Drawing for the job (mm, zero at the part's lowest x, y, z). A direction names the side the tool comes from. Give positions to 0.01 mm unless a question says otherwise; leave off trailing zeros. Loops run counter-clockwise (first coordinate to the right, second up) from the corner with the lowest first, then second, coordinate; pieces in that order, holes last. Notation, with made-up numbers: (-32.5, 12) - (2.5, 12) arc R37 cw to (2.5, 51) - close; hole circle Ø3 at (64.25, 51.5). An arc over 180 degrees is marked (long way). Return JSON: item names as keys, results as strings. Group by question number.
1) Slice it at A-A (y = 7.5). List the corners of the cut face in (x, z), and give its area (3 significant figures).
2) Drill centre lines: probe 1 along X at (y, z) = (6, 21); probe 2 along X at (y, z) = (2.2, 12.5); probe 3 along Y at (x, z) = (3, 14.5). Where is each one in solid material? Low to high. Write a range as from..to.
3) Slice it at C-C (x = 4.5). List the corners of the cut face in (y, z), and give its area (3 significant figures).
4) Slice it at D-D (y = 3.25). List the corners of the cut face in (x, z).
5) Drop a flat-ended pin along its axis: pin 1 (2.5 mm diameter, centred on x = 19, z = 12, fed in from +Y). Give the stop position or say it passes through.
6) Slice it at B-B (z = 12.5). List the corners of the cut face in (x, y).
7) 3-axis set-ups, long thin cutter, end or side, ignore diameter. For the marked faces 1 and 2: which of +Z, -Z, +X, -X, +Y, -Y reach the whole face in a straight line?
8) Mould opens along Z. For the marked faces 3, 4, 5 and 6 say: released by +Z, released by -Z, zero draft, split by the parting line, or undercut.
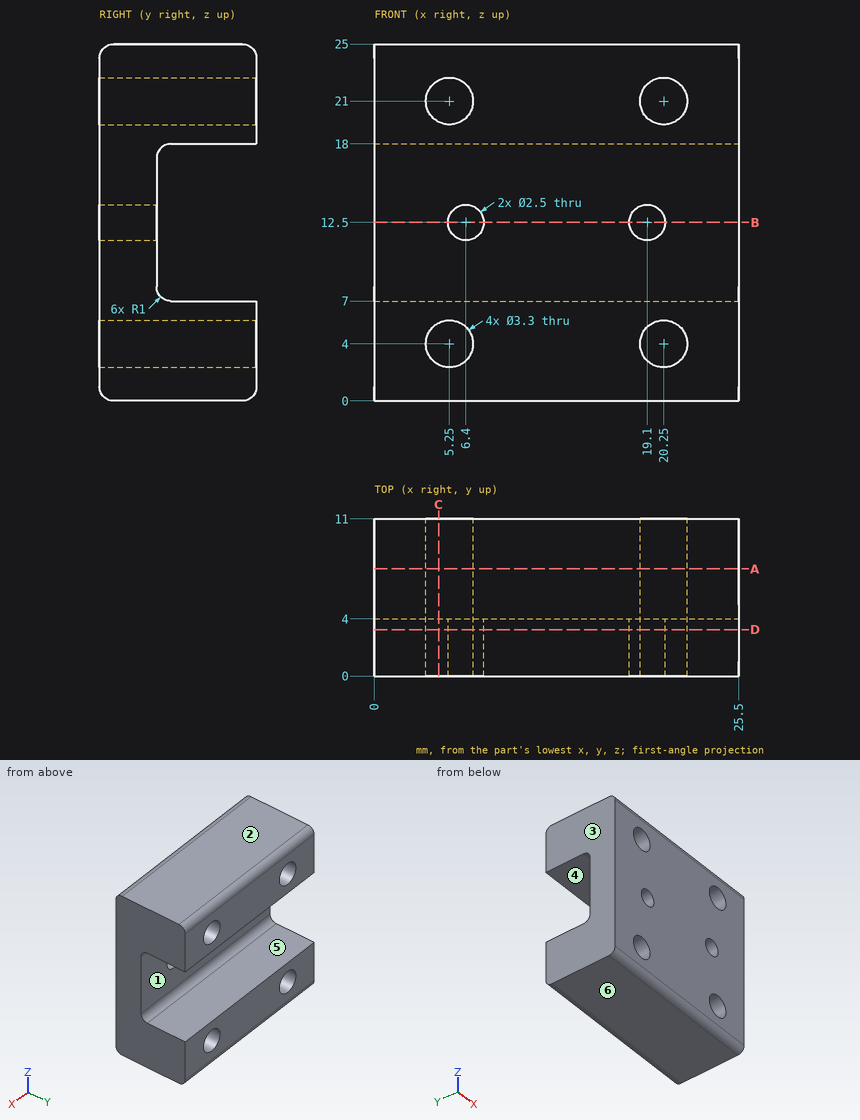
Results:
{
 "1": {"outline": "(0, 0) - (25.5, 0) - (25.5, 7) - (0, 7) - close; (0, 18) - (25.5, 18) - (25.5, 25) - (0, 25) - close; hole circle Ø3.3 at (5.25, 4); hole circle Ø3.3 at (5.25, 21); hole circle Ø3.3 at (20.25, 4); hole circle Ø3.3 at (20.25, 21)", "area": "323 mm2"},
 "2": {"probe 1": "0..3.6, 6.9..18.6, 21.9..25.5", "probe 2": "0..5.15, 7.65..17.85, 20.35..25.5", "probe 3": "0..4"},
 "3": {"outline": "(0, 1) arc R1 ccw to (1, 0) - (10, 0) arc R1 ccw to (11, 1) - (11, 2.53) - (0, 2.53) - close; (0, 5.47) - (11, 5.47) - (11, 7) - (5, 7) arc R1 cw to (4, 8) - (4, 17) arc R1 cw to (5, 18) - (11, 18) - (11, 19.53) - (0, 19.53) - close; (0, 22.47) - (11, 22.47) - (11, 24) arc R1 ccw to (10, 25) - (1, 25) arc R1 ccw to (0, 24) - close", "area": "133 mm2"},
 "4": {"outline": "(0, 0) - (25.5, 0) - (25.5, 25) - (0, 25) - close; hole circle Ø3.3 at (5.25, 4); hole circle Ø3.3 at (5.25, 21); hole circle Ø2.5 at (6.4, 12.5); hole circle Ø2.5 at (19.1, 12.5); hole circle Ø3.3 at (20.25, 4); hole circle Ø3.3 at (20.25, 21)"},
 "5": {"pin 1": "y = 4"},
 "6": {"outline": "(0, 0) - (5.15, 0) - (5.15, 4) - (0, 4) - close; (7.65, 0) - (17.85, 0) - (17.85, 4) - (7.65, 4) - close; (20.35, 0) - (25.5, 0) - (25.5, 4) - (20.35, 4) - close"},
 "7": {"face 1": "+X, -X, +Y", "face 2": "+Z, +X, -X, +Y, -Y"},
 "8": {"face 3": "zero draft", "face 4": "undercut", "face 5": "undercut", "face 6": "released by -Z"}
}
